Autodesk Fusion 360 part; units mm, degrees
sketch "Sketch1" plane through (0, 0, 0) normal (0, 1, 0) x (1, 0, 0)
  line L0 (0, 0) -> (95.5, 0)
  line L1 (95.5, 0) -> (95.5, 50)
  line L2 (95.5, 50) -> (0, 50)
  line L3 (0, 50) -> (0, 0)
  dimension "d1" = 95.5
  dimension "d2" = 50
extrude "Extrude1" add sketch "Sketch1" along normal blind 19
sketch "Sketch6" plane through (0, 19, 0) normal (0, 1, 0) x (-1, 0, 0)
  line L0 (0, -50) -> (0, 0)
  line L1 (0, 0) -> (-95.5, 0)
  line L2 (-95.5, 0) -> (-95.5, -50)
  line L3 (-95.5, -50) -> (0, -50)
  line L4 (-2, -2) -> (-93.5, -2)
  line L5 (-93.5, -2) -> (-93.5, -48)
  line L6 (-93.5, -48) -> (-2, -48)
  line L7 (-2, -48) -> (-2, -2)
  dimension "d39" = 91.5
  dimension "d40" = 46
extrude "Extrude5" cut sketch "Sketch6" against normal blind 17 contours L4 L5 L6 L7
sketch "Sketch8" plane through (0, 0, 0) normal (0, 0, 1) x (1, 0, 0)
  line L0 (0, 0) -> (95.5, 0)
  line L1 (95.5, 0) -> (95.5, 19)
  line L2 (95.5, 19) -> (0, 19)
  line L3 (0, 19) -> (0, 0)
  line L4 (0, 19) -> (42.5, 19)
  line L5 (42.5, 19) -> (42.5, 6)
  line L6 (42.5, 6) -> (0, 6)
  line L7 (0, 6) -> (0, 19)
  line L8 (42.5, 6) -> (52.9, 6)
  line L9 (52.9, 6) -> (52.9, 16)
  line L10 (52.9, 16) -> (42.5, 16)
  line L11 (42.5, 16) -> (42.5, 6)
  dimension "d66" = 42.5
  dimension "d67" = 13
  dimension "d68" = 10.4
  dimension "d69" = 10
extrude "Extrude7" cut sketch "Sketch8" against normal blind 2 contours L5 L8 L9 L10 L11
sketch "Sketch9" plane through (0, 0, -50) normal (0, 0, -1) x (-1, 0, 0)
  line L0 (-95.5, 0) -> (0, 0)
  line L1 (0, 0) -> (0, 19)
  line L2 (0, 19) -> (-95.5, 19)
  line L3 (-95.5, 19) -> (-95.5, 0)
  line L4 (-95.5, 19) -> (-51.5, 19)
  line L5 (-51.5, 19) -> (-51.5, 6)
  line L6 (-51.5, 6) -> (-95.5, 6)
  line L7 (-95.5, 6) -> (-95.5, 19)
  line L8 (-51.5, 6) -> (-64.5, 6)
  line L9 (-64.5, 6) -> (-64.5, 13.5)
  line L10 (-64.5, 13.5) -> (-51.5, 13.5)
  line L11 (-51.5, 13.5) -> (-51.5, 6)
  line L12 (-64.5, 6) -> (-72, 6)
  line L13 (-72, 6) -> (-72, 13.5)
  line L14 (-72, 13.5) -> (-64.5, 13.5)
  line L15 (-64.5, 13.5) -> (-64.5, 6)
  line L16 (-72, 6) -> (-85, 6)
  line L17 (-85, 6) -> (-85, 13.5)
  line L18 (-85, 13.5) -> (-72, 13.5)
  line L19 (-72, 13.5) -> (-72, 6)
  line L20 (-51.5, 6) -> (-44, 6)
  line L21 (-44, 6) -> (-44, 13.5)
  line L22 (-44, 13.5) -> (-51.5, 13.5)
  line L23 (-51.5, 13.5) -> (-51.5, 6)
  line L24 (-44, 6) -> (-31, 6)
  line L25 (-31, 6) -> (-31, 13.5)
  line L26 (-31, 13.5) -> (-44, 13.5)
  line L27 (-44, 13.5) -> (-44, 6)
  line L28 (-31, 6) -> (-23.5, 6)
  line L29 (-23.5, 6) -> (-23.5, 13.5)
  line L30 (-23.5, 13.5) -> (-31, 13.5)
  line L31 (-31, 13.5) -> (-31, 6)
  line L32 (-23.5, 6) -> (-10.5, 6)
  line L33 (-10.5, 6) -> (-10.5, 13.5)
  line L34 (-10.5, 13.5) -> (-23.5, 13.5)
  line L35 (-23.5, 13.5) -> (-23.5, 6)
  dimension "d72" = 44
  dimension "d73" = 13
  dimension "d74" = 13
  dimension "d75" = 7.5
  dimension "d76" = 7.5
  dimension "d77" = 7.5
  dimension "d78" = 13
  dimension "d79" = 7.5
  dimension "d80" = 7.5
  dimension "d81" = 7.5
  dimension "d82" = 13
  dimension "d83" = 7.5
  dimension "d84" = 7.5
  dimension "d85" = 7.5
  dimension "d86" = 13
  dimension "d87" = 7.5
extrude "Extrude8" cut sketch "Sketch9" against normal blind 2 contours L6 L13 L16 L17 L18 L19 | L5 L6 L8 L9 L10 L11 L15 L23 | L21 L24 L25 L26 L27 L31 | L29 L32 L33 L34 L35
sketch "Sketch10" plane through (0, 0, 0) normal (0, 1, 0) x (1, 0, 0)
  line L0 (2, 2) -> (5.75, 2)
  line L1 (5.75, 2) -> (5.75, 5.5)
  line L2 (5.75, 5.5) -> (2, 5.5)
  line L3 (2, 5.5) -> (2, 2)
  circle A0 centre (5.75, 5.5) radius 3
  line L4 (2, 48) -> (5.75, 48)
  line L5 (5.75, 48) -> (5.75, 44.5)
  line L6 (5.75, 44.5) -> (2, 44.5)
  line L7 (2, 44.5) -> (2, 48)
  circle A1 centre (5.75, 44.5) radius 3
  line L8 (93.5, 48) -> (89.75, 48)
  line L9 (89.75, 48) -> (89.75, 44.5)
  line L10 (89.75, 44.5) -> (93.5, 44.5)
  line L11 (93.5, 44.5) -> (93.5, 48)
  circle A2 centre (89.75, 44.5) radius 3
  line L12 (93.5, 2) -> (89.75, 2)
  line L13 (89.75, 2) -> (89.75, 5.5)
  line L14 (89.75, 5.5) -> (93.5, 5.5)
  line L15 (93.5, 5.5) -> (93.5, 2)
  circle A3 centre (89.75, 5.5) radius 3
  dimension "d93" = 3.75
  dimension "d94" = 3.5
  dimension "d95" = 6
  dimension "d96" = 3.75
  dimension "d97" = 3.5
  dimension "d98" = 6
  dimension "d99" = 3.75
  dimension "d100" = 3.5
  dimension "d101" = 6
  dimension "d102" = 3.75
  dimension "d103" = 3.5
  dimension "d104" = 6
extrude "Extrude9" add sketch "Sketch10" along normal blind 5 contours L1 L2 A0 | L1 L2 A0 | L5 L6 A1 | L5 L6 A1 | L9 L10 A2 | L9 L10 A2 | L13 L14 A3 | L13 L14 A3
hole "Hole5" at (5.75, 5, -44.5) direction (0, -1, 0) diameter 2.529 depth 5 tip angle 180
hole "Hole6" at (89.75, 5, -44.5) direction (0, -1, 0) diameter 2.529 depth 5 tip angle 180
hole "Hole7" at (89.75, 5, -5.5) direction (0, -1, 0) diameter 2.529 depth 5 tip angle 180
hole "Hole8" at (5.75, 5, -5.5) direction (0, -1, 0) diameter 2.529 depth 5 tip angle 180
Here's how the part is built. I have some questions about the finished solid (model axes, mm). A direction names the side the tool comes from. Coordinates: 2 decimals unless noted, no trailing zeros. Write each loop counter-clockwise with the first axis right and the second up, starting at its lowest first coordinate (ties: lowest second). Pieces come first, ordered by that corner, then holes.
1) Thinking about a two-plate mould opening in Z: for faces 4 (the face through (6, 5, -4)), 5 (the face through (64.5, 10, -49)), 6 (the face through (48, 9, -50)), 7 (the face through (93.5, 11, -25)), which applies, +Z half, -Z half, draft (parallel to the pull), parting line (faces both ways), or undercut?
Filled in:
face 4: undercut
face 5: draft
face 6: -Z half
face 7: undercut
2) Which directions (+Z, -Z, +X, -X, +Y, -Y) give clear straight access to the entire face, cutting with the end or side of a thin tool? Please do faces 1 (the face through (52.9, 11, -1)), 2 (the face through (58, 13.5, -49)), 3 (the face through (90, 5, -43)).
Filled in:
face 1: +Z
face 2: -Z
face 3: +Y
3) If we section it at D-D (x = 79): List the corners of the cut face in (y, z) for me.
Filled in:
outline: (0, -50) - (6, -50) - (6, -48) - (2, -48) - (2, -2) - (19, -2) - (19, 0) - (0, 0) - close; (13.5, -50) - (19, -50) - (19, -48) - (13.5, -48) - close
4) If we section it at C-C (z = -5.5): List the corners of the cut face in (x, y) for me, plus the area to 3 significant figures.
Filled in:
outline: (0, 0) - (4.49, 0) - (4.49, 5) - (2.75, 5) - (2.75, 2) - (2, 2) - (2, 19) - (0, 19) - close; (7.01, 0) - (88.49, 0) - (88.49, 5) - (86.75, 5) - (86.75, 2) - (8.75, 2) - (8.75, 5) - (7.01, 5) - close; (91.01, 0) - (95.5, 0) - (95.5, 19) - (93.5, 19) - (93.5, 2) - (92.75, 2) - (92.75, 5) - (91.01, 5) - close
area: 270 mm2
5) If we section it at B-B (x = 89.75): List the corners of the cut face in (y, z) for me.
Filled in:
outline: (0, -50) - (19, -50) - (19, -48) - (2, -48) - (2, -47.5) - (5, -47.5) - (5, -45.76) - (0, -45.76) - close; (0, -43.24) - (5, -43.24) - (5, -41.5) - (2, -41.5) - (2, -8.5) - (5, -8.5) - (5, -6.76) - (0, -6.76) - close; (0, -4.24) - (5, -4.24) - (5, -2.5) - (2, -2.5) - (2, -2) - (19, -2) - (19, 0) - (0, 0) - close
6) I'm going to push flat-ended pins straight in: pin 1 (3 mm diameter, centred on x = 53.5, z = -42.5, fed in from +Y); pin 2 (6.5 mm diameter, centred on x = 88.5, z = -6.5, fed in from +Y). Where does each tip first touch, or does it pass through?
Filled in:
pin 1: stops at y = 2
pin 2: stops at y = 5
7) If I drill on line 1 (X direction, y = 1.7, z = -5.5); line 2 (Z direction, x = 5.75, y = 2.1); line 3 (Z direction, x = 5.75, y = 1.2), over which ranges is the centre line in solid material (lowest first)?
Filled in:
line 1: x = 0 to 4.49, 7.01 to 88.49, 91.01 to 95.5
line 2: z = -50 to -48, -47.5 to -45.76, -43.24 to -41.5, -8.5 to -6.76, -4.24 to -2.5, -2 to 0
line 3: z = -50 to -45.76, -43.24 to -6.76, -4.24 to 0
8) If we section it at A-A (y = 3.5): Count the separate pieces of the cut face and the enclosed holes in it, plus the area to 3 significant figures.
Filled in:
separate pieces: 5
enclosed holes: 5
area: 659 mm2
